CAD build for the part. Positions are in the model's coordinates, mm. A direction names the side the tool comes from. Coordinates: 2 decimals unless noted, no trailing zeros. Order: outer loops, then holes, each group sorted by start corner. A loop starts at its lowest first (then second) coordinate and runs counter-clockwise, first axis right, second up.
from build123d import *

# Parameters (mm, degrees)
SKETCH1_R           = 14.3891
SKETCH1_R_2         = 5.9309
BOSS_EXTRUDE2_DEPTH = 6.35
SKETCH2_R           = 2.413
CUT_EXTRUDE1_DEPTH  = 6.35
CUT_EXTRUDE6_START  = -6.35
CUT_EXTRUDE6_DEPTH  = 6.35
FILLET4_R           = 3.175
FILLET6_R           = 3.175
FILLET5_R           = 3.175


# Read off the part's stored shape, not the designer's step: Cut-Extrude6
with BuildPart() as part:
    # Sketch1 → Boss-Extrude2 (new body)
    with BuildSketch(Plane.XY):
        with BuildLine():
            Line((-50.700880407, 49.587781591), (54.963119593, 49.587781591))
            ThreePointArc((54.963119593, 49.587781591), (63.943375714, 45.868037712), (67.663119593, 36.887781591))
            Line((67.663119593, 36.887781591), (67.663119593, -43.122218409))
            ThreePointArc((67.663119593, -43.122218409), (63.943375714, -52.10247453), (54.963119593, -55.822218409))
            Line((54.963119593, -55.822218409), (-50.700880407, -55.822218409))
            ThreePointArc((-50.700880407, -55.822218409), (-59.681136528, -52.10247453), (-63.400880407, -43.122218409))
            Line((-63.400880407, -43.122218409), (-63.400880407, 36.887781591))
            ThreePointArc((-63.400880407, 36.887781591), (-59.681136528, 45.868037712), (-50.700880407, 49.587781591))
        make_face()
        Circle(SKETCH1_R, mode=Mode.SUBTRACT)
        with Locations((35.939214506, -24.072218409)):
            Circle(SKETCH1_R, mode=Mode.SUBTRACT)
        with Locations((32.791546632, 16.934641063)):
            Circle(SKETCH1_R_2, mode=Mode.SUBTRACT)
        with Locations((-32.69260882, 17.124862832)):
            Circle(SKETCH1_R_2, mode=Mode.SUBTRACT)
    extrude(amount=BOSS_EXTRUDE2_DEPTH)

    # Sketch2 → Cut-Extrude1 (cut)
    with BuildSketch(Plane.XY.offset(6.35)):
        with Locations((-50.700880407, 36.887781591)):
            Circle(SKETCH2_R)
        with Locations(Location((54.963119593, 36.887781591, 0), (0, 0, 180))):
            Circle(SKETCH2_R)
        with Locations((54.963119593, -43.122218409)):
            Circle(SKETCH2_R)
        with Locations(Location((-50.700880407, -43.122218409, 0), (0, 0, 180))):
            Circle(SKETCH2_R)
    extrude(amount=-CUT_EXTRUDE1_DEPTH, mode=Mode.SUBTRACT)

    # Cut-Extrude6 outline → Cut-Extrude6 (cut)
    with BuildSketch(Plane.XY.offset(6.35).offset(CUT_EXTRUDE6_START)):
        with BuildLine():
            ThreePointArc((-22.865276921, 20.166764197), (-1.620277869, 30.444933347), (20.595631427, 22.479751622))
            ThreePointArc((20.595631427, 22.479751622), (26.18341036, 28.588873504), (34.294760977, 30.247377274))
            Line((34.294760977, 30.247377274), (44.495862095, 39.427781591))
            Line((44.495862095, 39.427781591), (-45.782707456, 39.427781591))
            Line((-45.782707456, 39.427781591), (-34.660782298, 27.22218472))
            ThreePointArc((-34.660782298, 27.22218472), (-27.411857693, 25.953412186), (-22.865276921, 20.166764197))
        make_face()
        with BuildLine():
            ThreePointArc((12.980930477, -27.58649508), (-15.657094436, -26.160555435), (-30.44625116, -1.595323538))
            ThreePointArc((-30.44625116, -1.595323538), (-41.465480232, 4.60457782), (-53.240880407, 0))
            Line((-53.240880407, 0), (-53.240880407, -35.100222849))
            ThreePointArc((-53.240880407, -35.100222849), (-44.750921888, -37.17225989), (-42.678884848, -45.662218409))
            Line((-42.678884848, -45.662218409), (27.37738958, -45.662218409))
            ThreePointArc((27.37738958, -45.662218409), (17.771598796, -38.541865449), (12.980930477, -27.58649508))
        make_face()
        with BuildLine():
            ThreePointArc((46.188533959, 17.031229414), (44.21986427, 9.94306365), (38.805433181, 4.962934111))
            Line((38.805433181, 4.962934111), (39.269790063, -1.08656609))
            ThreePointArc((39.269790063, -1.08656609), (50.308421041, -5.825058365), (57.503119593, -15.444881422))
            Line((57.503119593, -15.444881422), (57.503119593, 27.213705757))
            Line((57.503119593, 27.213705757), (46.188533959, 17.031229414))
        make_face()
    extrude(amount=CUT_EXTRUDE6_DEPTH, mode=Mode.SUBTRACT)

    # Fillet4
    fillet4_edges = [part.edges().sort_by_distance(p)[0] for p in [
        (39.269790063, -1.08656609, 3.175),
        (-22.865276921, 20.166764197, 3.175),
        (-34.660782298, 27.22218472, 3.175),
        (-45.782707456, 39.427781591, 3.175),
        (44.495862095, 39.427781591, 3.175),
        (34.294760977, 30.247377274, 3.175),
        (46.188533959, 17.031229414, 3.175),
        (57.503119593, 27.213705757, 3.175),
        (57.503119593, -15.444881422, 3.175),
    ]]
    fillet(fillet4_edges, radius=FILLET4_R)

    # Fillet6
    fillet6_edges = [part.edges().sort_by_distance(p)[0] for p in [
        (20.595631427, 22.479751622, 3.175),
    ]]
    fillet(fillet6_edges, radius=FILLET6_R)

    # Fillet5
    fillet5_edges = [part.edges().sort_by_distance(p)[0] for p in [
        (-42.678884848, -45.662218409, 3.175),
        (-53.240880407, -35.100222849, 3.175),
        (-53.240880407, 0, 3.175),
        (-30.44625116, -1.595323538, 3.175),
        (12.980930477, -27.58649508, 3.175),
        (27.37738958, -45.662218409, 3.175),
    ]]
    fillet(fillet5_edges, radius=FILLET5_R)


solid = part.part
1) Drill centre lines: probe 1 along Y at (x, z) = (0, 3.75); probe 2 along Y at (x, z) = (-38, 3.5); probe 3 along Y at (x, z) = (24, 1). Where is each one in solid material? Low to high.
2) Two-plate mould, pull along Y, no slides. Class faces 1 (the flat face through (18, -2, 6.35)), 2 (the cylindrical face through (64.042, -52.003, 3.131)), 3 (the cylindrical face through (47.121, -3.715, 3.131)), 4 (the cylindrical face through (55.613, -8.033, 3.219)): released by +Y, released by -Y, zero draft, split by the parting line, or undercut.
3) Which spindle directions (+Z, -Z, +X, -X, +Y, -Y) get a long thin tool onto all of the face, cutting with end or side? Do faces 5 (the cylindrical face through (-59.58, -52.2, 3.13)), 6 (the flat face through (-53.241, -16, 3)). Say none if no direction does.
4) Slice it at C-C (z = 4). Give the number of separate pieces and of enclosed holes in the cut face, plus the area to 3 significant figures.
5) Slice it at A-A (x = 0). List the corners of the cut face in (y, z).
6) Slice it at B-B (x = 31.5). List the corners of the cut face in (y, z), plus the area to 3 significant figures.
Worked out:
1. probe 1: y = -55.82 to -45.66, -30.49 to -14.39, 14.39 to 30.49, 39.43 to 49.59
1. probe 2: y = -55.82 to -45.66, 3.94 to 14.48, 19.77 to 30.89, 39.43 to 49.59
1. probe 3: y = -55.82 to -32.1, -16.04 to 27.04, 39.43 to 49.59
2. face 1: zero draft
2. face 2: released by -Y
2. face 3: undercut
2. face 4: undercut
3. face 5: +Z, -Z, -X, -Y
3. face 6: +Z, -Z
4. separate pieces: 1
4. enclosed holes: 11
4. area: 8,860 mm2
5. outline: (-55.82, 0) - (-45.66, 0) - (-45.66, 6.35) - (-55.82, 6.35) - close; (-30.49, 0) - (-14.39, 0) - (-14.39, 6.35) - (-30.49, 6.35) - close; (14.39, 0) - (30.49, 0) - (30.49, 6.35) - (14.39, 6.35) - close; (39.43, 0) - (49.59, 0) - (49.59, 6.35) - (39.43, 6.35) - close
6. outline: (-55.82, 0) - (-37.76, 0) - (-37.76, 6.35) - (-55.82, 6.35) - close; (-10.39, 0) - (11.15, 0) - (11.15, 6.35) - (-10.39, 6.35) - close; (22.72, 0) - (30.27, 0) - (30.27, 6.35) - (22.72, 6.35) - close; (39.43, 0) - (49.59, 0) - (49.59, 6.35) - (39.43, 6.35) - close
6. area: 364 mm2
